Verification items for the finished model (mm, model axes). A direction names the side the tool comes from. Coordinates: 2 decimals unless noted, no trailing zeros. Write each loop counter-clockwise with the first axis right and the second up, starting at its lowest first coordinate (ties: lowest second). Pieces come first, ordered by that corner, then holes. Notation, with made-up numbers: (33.25, 15) - (63.25, 15) arc R12 cw to (63.25, 20) - close; hole circle Ø10 at (11.25, 79.25). An arc over 180 degrees is marked (long way). Use one line per item in the form item = value. Start each with the question number.
(1) Sectioned sample at A-A (x = 0). Record the cut outline in (y, z), and give its area (3 significant figures).
(2) Tool access check on faces 5 (the conical face through (14.946, 4.707, 101.225)), 6 (the cylindrical face through (12.39, -55.78, 12.52)). Record the directions out of +Z, -Z, +X, -X, +Y, -Y that give a thin tool (end or side, any length) a straight path to the whole face; none if there is none.
(3) Gauge pin test, flat ends, axial feed: pin 1 Ø1 at (y, z) = (7, 77.5) entering from -X; pin 2 Ø1.5 at (x, z) = (-17.5, 57) entering from -Y; pin 3 Ø6 at (y, z) = (27, 20.5) entering from +X; pin 4 Ø3 at (x, y) = (-1, -19) entering from -Z. Record the tip position at first contact, or that the pin passes through.
(4) Mould release check, pull along Z, two halves, no side actions. Record for faces 1 (the flat face through (1, 1, 0)), 2 (the conical face through (12.23, 3.85, 143.82)), 3 (the cylindrical face through (12.871, -4.053, 157.752)), 4 (the flat face through (0, 0, 164.191)): released by +Z, released by -Z, zero draft, split by the parting line, or undercut.
(5) Sectioned sample at C-C (z = 57). Record the cut outline in (x, y).
(6) Material ranges on line 1 (X direction, y = -10.5, z = 32); line 2 (Y direction, x = -3.5, z = 157); line 3 (Z direction, x = -26.5, y = -43.5), recorded low to high. Write a range as [from, to].
(7) Sectioned sample at B-B (z = 112.5). Record the cut outline in (x, y), and give its area (3 significant figures).
from build123d import *

# Parameters (mm, degrees)
F1_FACE_R = 19.05
F2_DEPTH  = 76.2
F2_TAPER  = 5
F2_FACE_R = 12.3833638393
F3_DEPTH  = 12.7
F3_TAPER  = -5
F4_DEPTH  = 12.7


with BuildPart() as f1:
    # F0 (on Front) → F1 (revolve)
    with BuildSketch(Plane.XZ):
        with BuildLine():
            Line((-57.1391619384, 0), (0, 0))
            Line((0, 0), (0, 62.5912960728))
            Line((0, 62.5912960728), (-19.05, 62.5912960728))
            ThreePointArc((-19.05, 62.5912960728), (-30.5216077648, 36.2398494169), (-57.1391619384, 25.4))
            Line((-57.1391619384, 25.4), (-57.1391619384, 0))
        make_face()
    revolve(axis=Axis((0, 0, 31.2956480364), (0, 0, -1)))

    # F1_face (on face) → F2 (join)
    with BuildSketch(Plane.XY.offset(62.5912960728)):
        Circle(F1_FACE_R)
    extrude(amount=F2_DEPTH, taper=F2_TAPER)

    # F2_face (on face) → F3 (join)
    with BuildSketch(Plane.XY.offset(138.7912960728)):
        Circle(F2_FACE_R)
    extrude(amount=F3_DEPTH, taper=F3_TAPER)

    # F4 (add): a face of the model
    f4_faces = [f1.faces().sort_by_distance(p)[0] for p in [
        (0, 0, 151.4912960728),
    ]]
    extrude(f4_faces, amount=F4_DEPTH)


solid = f1.part
Answers below:
q1.outline = (-57.14, 0) - (57.14, 0) - (57.14, 25.4) arc R38.1 cw to (19.05, 62.59) - (12.38, 138.79) - (13.49, 151.49) - (13.49, 164.19) - (-13.49, 164.19) - (-13.49, 151.49) - (-12.38, 138.79) - (-19.05, 62.59) arc R38.1 cw to (-57.14, 25.4) - close
q1.area = 8,010 mm2
q2.face_5 = none
q2.face_6 = +Z, -Z
q3.pin_1 = -16.52
q3.pin_2 = -10.2
q3.pin_3 = 51.85
q3.pin_4 = 0
q4.face_1 = released by -Z
q4.face_2 = undercut
q4.face_3 = zero draft
q4.face_4 = released by +Z
q5.outline = circle Ø39.2 at (0, 0)
q6.line_1 = [-34.13, 34.13]
q6.line_2 = [-13.03, 13.03]
q6.line_3 = [0, 25.91]
q7.outline = circle Ø29.37 at (0, 0)
q7.area = 677 mm2
